Check sheet for the modelled part. Datum: model origin and axes. Units: mm. A direction names the side the tool comes from. Round coordinates to 2 decimals unless told otherwise and drop trailing zeros. Write each loop counter-clockwise with the first axis right and the second up, starting at its lowest first coordinate (ties: lowest second). Pieces come first, ordered by that corner, then holes.
Item 1: Section check B-B, the plane x = 105. Record the cut outline in (y, z).
Item 2: Section check C-C, the plane y = 79. Record the cut outline in (x, z).
Item 3: Material ranges on line 1 along Z through (x, y) = (75, 29); line 2 along X through (y, z) = (31, 74.5); line 3 along Y through (x, z) = (83.5, 111), recorded low to high.
Item 4: Section check A-A, the plane z = 74.5. Record the cut outline in (x, y), plus the area to 3 significant figures.
Item 5: Depth check by flat-ended pin: pin 1 (5 mm diameter, centred on x = 49, y = 62.5, fed in from +Z); pin 2 (8 mm diameter, centred on y = 55, z = 74.5, fed in from -X); pin 3 (6 mm diameter, centred on x = 59.5, y = 59.5, fed in from -Z). Enter the tip coordinate at first touch or a pass-through.
Item 6: Set-up check for faces 1 (the cylindrical face through (115.645, 40.426, 91.352)), 2 (the flat face through (75, 2.5, 122)), 3 (the flat face through (30.7, 0, 74.2)): record each of +Z, -Z, +X, -X, +Y, -Y from which the full face is reachable in a straight line by a thin tool's end or side.
from build123d import *

# Parameters (mm, degrees)
CYLINDER020_R             = 44
CYLINDER020_DEPTH         = 2.5
CYLINDER018_R             = 54
CYLINDER018_DEPTH         = 2.5
CYLINDER019_R             = 44
CYLINDER019_DEPTH         = 79.5
CYLINDER017_R             = 47.25
CYLINDER017_DEPTH         = 81.5
FUSION004_PLACEMENT_ANGLE = 90


with BuildPart() as cylinder016:
    # Cylinder020 → Cylinder020 (new body)
    with BuildSketch(Plane.XY.offset(-2.5)):
        Circle(CYLINDER020_R)
    extrude(amount=CYLINDER020_DEPTH)


with BuildPart() as cut004003:
    # Cylinder018 → Cylinder018 (new body)
    with BuildSketch(Plane.XY.offset(-2.5)):
        Circle(CYLINDER018_R)
    extrude(amount=CYLINDER018_DEPTH)

    # Cut004003: cut Cylinder016
    add(cylinder016.part, mode=Mode.SUBTRACT)


with BuildPart() as cylinder015:
    # Cylinder019 → Cylinder019 (new body)
    with BuildSketch(Plane.XY):
        Circle(CYLINDER019_R)
    extrude(amount=CYLINDER019_DEPTH)


with BuildPart() as cup:
    # Cylinder017 → Cylinder017 (new body)
    with BuildSketch(Plane.XY):
        Circle(CYLINDER017_R)
    extrude(amount=CYLINDER017_DEPTH)

    # Cut004002: cut Cylinder015
    add(cylinder015.part, mode=Mode.SUBTRACT)

    # Fusion004: union Cut004003
    add(cut004003.part)


with BuildPart() as cup_1:
    # Fusion004 placement: moved
    add(cup.part.moved(Location((75, 2.5, 74.5))).rotate(Axis((75, 2.5, 74.5), (-1, 0, 0)), FUSION004_PLACEMENT_ANGLE))


solid = cup_1.part
Values found:
1. outline: (0, 29.6) - (2.5, 29.6) - (2.5, 38) - (84, 38) - (84, 111) - (2.5, 111) - (2.5, 119.4) - (0, 119.4) - (0, 106.69) - (82, 106.69) - (82, 42.31) - (0, 42.31) - close
2. outline: circle Ø94.5 at (75, 74.5); hole circle Ø88 at (75, 74.5)
3. line 1: z = 27.25 to 30.5, 118.5 to 121.75
3. line 2: x = 27.75 to 31, 119 to 122.25
3. line 3: y = 82 to 84
4. outline: (21, 0) - (31, 0) - (31, 82) - (119, 82) - (119, 0) - (129, 0) - (129, 2.5) - (122.25, 2.5) - (122.25, 84) - (27.75, 84) - (27.75, 2.5) - (21, 2.5) - close
4. area: 756 mm2
5. pin 1: stops at z = 115.49
5. pin 2: stops at x = 27.75
5. pin 3: stops at z = 28.93
6. face 1: -Y
6. face 2: +Y
6. face 3: +Z, -Z, +X, -X, -Y
